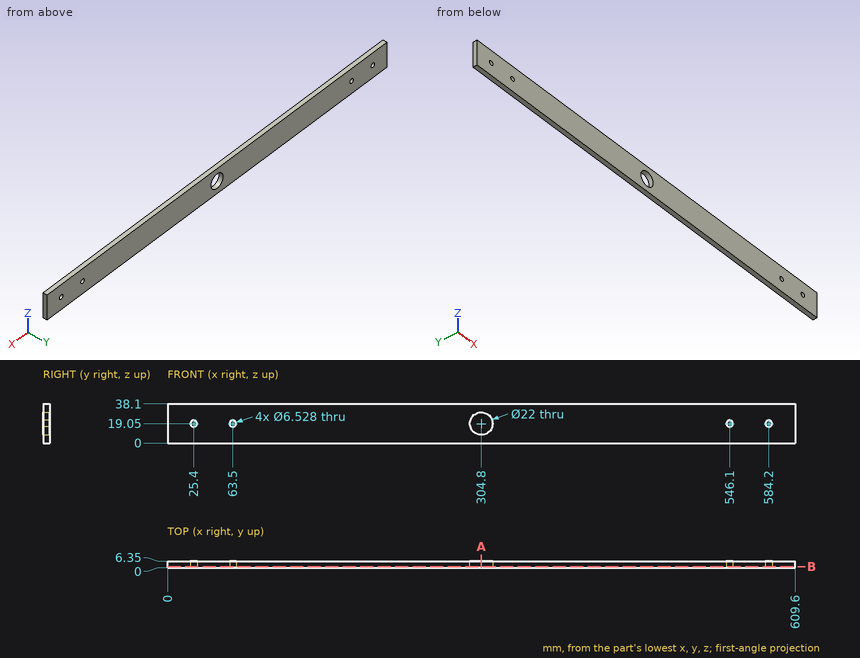
Drawing for the job (mm, zero at the part's lowest x, y, z). Round coordinates to 2 decimals unless told otherwise and drop trailing zeros. Loops run counter-clockwise (first coordinate to the right, second up) from the corner with the lowest first, then second, coordinate; pieces in that order, holes last. Notation, with made-up numbers: (-14, 32) - (19, 32) arc R22 ccw to (19, 52) - close; hole circle Ø6 at (56, 84). An arc over 180 degrees is marked (long way). Return JSON: item names as keys, results as strings. Group by question number.
Q1. Band-saw the part on A-A on x = 304.8. Give the cut face in (y, z), plus the area to 3 significant figures.
Q2. Drill centre lines: line 1 along Z through (x, y) = (584.2, 2.25); line 2 along X through (y, z) = (3.5, 29); line 3 along X through (y, z) = (3.25, 15). Where is each one in solid material? Low to high. Write a range as [from, to].
Q3. Flat gauge pin, fed straight in: pin 1 Ø10.5 at (x, z) = (546.1, 19.05) entering from +Y. Where does the tip first touch, or does it go through?
Q4. Band-saw the part on B-B on y = 1. Give the cut face in (x, z), plus the area to 3 significant figures.
Solutions:
{
 "1": {"outline": "(0, 0) - (6.35, 0) - (6.35, 8.05) - (0, 8.05) - close; (0, 30.05) - (6.35, 30.05) - (6.35, 38.1) - (0, 38.1) - close", "area": "102 mm^2"},
 "2": {"line 1": "z = [0, 15.79], [22.31, 38.1]", "line 2": "x = [0, 300.11], [309.49, 609.6]", "line 3": "x = [0, 294.57], [315.03, 609.6]"},
 "3": {"pin 1": "stops at y = 6.35"},
 "4": {"outline": "(0, 0) - (609.6, 0) - (609.6, 38.1) - (0, 38.1) - close; hole circle Ø6.53 at (25.4, 19.05); hole circle Ø6.53 at (63.5, 19.05); hole circle Ø22 at (304.8, 19.05); hole circle Ø6.53 at (546.1, 19.05); hole circle Ø6.53 at (584.2, 19.05)", "area": "22,700 mm^2"}
}
